Source: CAD feature listing. Evaluate the final solid. Frame: model axes, mm. A direction names the side the tool comes from. Round coordinates to 2 decimals unless told otherwise and drop trailing zeros. Loops run counter-clockwise (first coordinate to the right, second up) from the corner with the lowest first, then second, coordinate; pieces in that order, holes last. Notation, with made-up numbers: (6.25, 65.25) -> (62.25, 65.25) arc R20 ccw to (62.25, 77.25) -> close; hole circle Ø6 at (32.5, 89). An arc over 180 degrees is marked (long way). Put each result on its own line as item: value. Start each with the question number.
1. Material intervals for L1, parallel to X at y = 98, z = 17; L2, parallel to Y at x = 15, z = 1.2; L3, parallel to Z at x = 19, y = 74, sorted ascending.
2. Set-up query: faces 1 (the cylindrical face through (0, 81, 10)), 2 (the flat face through (22.9, 72.35, 1.48)), 3 (the flat face through (-22.956, 72.567, 1.479)), 4 (the cylindrical face through (20.91, 85.2, 16.48)), 5 (the cylindrical face through (14.979, 108.449, 4.725)). Return all of +Z, -Z, +X, -X, +Y, -Y with unobstructed straight access to the full face (end or side cutting, diameter ignored); none if empty.
3. Cut plane C-C (x = -2.5). State how many separate pieces and enclosed holes the cut face has, then the cut area to 3 significant figures.
4. Draft query along Y for faces 6 (the flat face through (0, 111, 15.5)), 7 (the flat face through (24.547, 78.741, 8.916)), 8 (the cylindrical face through (6.693, 109.541, 7.371)). Return one class per face: pulls with the +Y half, pulls with the -Y half, needs draft (parallel to the pull), parting line crosses it, or undercut.
5. Cut plane B-B (y = 82). Return the cut outline in (x, z).
6. Cut plane A-A (z = 8.25). Return the cut outline in (x, y), then the cut area to 3 significant figures.
7. Contact query for flat-ended pins moving along their axis: pin 1 (8 mm diameter, centred on x = 4, y = 70, fed in from +Z); pin 2 (2.5 mm diameter, centred on x = -0.5, y = 110.5, fed in from +Z); pin 3 (6 mm diameter, centred on x = 0, z = 8.25, fed in from -Y). Output: stop coordinate, or through.
```python
from build123d import *

# Parameters (mm, degrees)
SKETCH1_R                 = 2
BOSS_EXTRUDE1_DEPTH       = 3
BOSS_EXTRUDE2_DEPTH       = 12
SKETCH3_R                 = 1.5
BOSS_EXTRUDE3_DEPTH       = 3
FILLET1_R                 = 10
FILLET3_R                 = 3.5
BOSS_EXTRUDE6_DEPTH       = 14
BOSS_EXTRUDE7_DEPTH       = 0.5
BOSS_EXTRUDE8_START       = -14
BOSS_EXTRUDE8_DEPTH       = 14
FILLET7_R                 = 30
FILLET11_R                = 30
CUT_EXTRUDE3_REACH        = 52.603
CUT_EXTRUDE3_END_RADIUS   = 47
SKETCH12_R                = 3.75
BOSS_EXTRUDE9_REACH       = 64
BOSS_EXTRUDE9_END_RADIUS  = 47
SKETCH13_R                = 6.75
SKETCH13_R_2              = 3.75
BOSS_EXTRUDE10_REACH      = 59.242
BOSS_EXTRUDE10_END_RADIUS = 44
SKETCH14_R                = 6.75
SKETCH14_R_2              = 3.75


# Some blends are built 0.0001 mm under size
with BuildPart() as part:
    # Sketch1 → Boss-Extrude1 (new body)
    with BuildSketch(Plane.XY):
        with BuildLine():
            Line((20.854716842, 64.723108589), (25, 80.193515947))
            ThreePointArc((25, 80.193515947), (0, 84), (-25, 80.193515947))
            Line((-25, 80.193515947), (-20.854716842, 64.723108589))
            ThreePointArc((-20.854716842, 64.723108589), (0, 68), (20.854716842, 64.723108589))
        make_face()
        with Locations((15, 70.420167566)):
            Circle(SKETCH1_R, mode=Mode.SUBTRACT)
        with Locations(Location((-15, 70.420167566, 0), (0, 0, 180))):
            Circle(SKETCH1_R, mode=Mode.SUBTRACT)
    extrude(amount=BOSS_EXTRUDE1_DEPTH)

    # Sketch2 → Boss-Extrude2 (add)
    with BuildSketch(Plane.XY.offset(3)):
        with BuildLine():
            Line((-25, 80.193515947), (-24.107142857, 77.329461806))
            ThreePointArc((-24.107142857, 77.329461806), (0, 81), (24.107142857, 77.329461806))
            Line((24.107142857, 77.329461806), (25, 80.193515947))
            ThreePointArc((25, 80.193515947), (0, 84), (-25, 80.193515947))
        make_face()
    extrude(amount=BOSS_EXTRUDE2_DEPTH)

    # Sketch3 → Boss-Extrude3 (add)
    with BuildSketch(Plane.XY.offset(15)):
        with BuildLine():
            Line((-31.5, 77.329461806), (-31.5, 105.329461806))
            Line((-31.5, 105.329461806), (-24.5, 105.329461806))
            Line((-24.5, 105.329461806), (-24.5, 80.347681983))
            ThreePointArc((-24.5, 80.347681983), (0, 84), (24.5, 80.347681983))
            Line((24.5, 80.347681983), (24.5, 105.329461806))
            Line((24.5, 105.329461806), (31.5, 105.329461806))
            Line((31.5, 105.329461806), (31.5, 77.329461806))
            Line((31.5, 77.329461806), (24.107142857, 77.329461806))
            ThreePointArc((24.107142857, 77.329461806), (0, 81), (-24.107142857, 77.329461806))
            Line((-24.107142857, 77.329461806), (-31.5, 77.329461806))
        make_face()
        with Locations((-28, 101.920167566)):
            Circle(SKETCH3_R, mode=Mode.SUBTRACT)
        with Locations(Location((28, 101.920167566, 0), (0, 0, 180))):
            Circle(SKETCH3_R, mode=Mode.SUBTRACT)
    extrude(amount=BOSS_EXTRUDE3_DEPTH)

    # Fillet1
    # the kernel refuses this fillet: 10 mm, written as the material it adds along each edge
    with BuildSketch(Plane(origin=(24.5, 80.347681983, 15), x_dir=(-0.9747000358663407, 0.22351697940459464, 0), z_dir=(0, 0, 1))) as fillet1_piece_1:
        with BuildLine():
            CenterArc((12.54704984, -9.975125536), FILLET1_R, 94.042076765, 98.87360977)
            Line((2.800049481, -12.21029533), (0, 0))
            ThreePointArc((0, 0), (5.9210797, -0.208945494), (11.8421594, 0))
        make_face()
    extrude(amount=3)
    with BuildSketch(Plane(origin=(-24.5, 80.347681983, 15), x_dir=(0.9747000358663402, 0.22351697940459697, 0), z_dir=(0, 0, 1))) as fillet1_piece_2:
        with BuildLine():
            CenterArc((12.54704984, 9.975125536), FILLET1_R, 167.084313465, 98.87360977)
            Line((2.800049481, 12.21029533), (0, 0))
            ThreePointArc((0, 0), (5.9210797, 0.208945494), (11.8421594, 0))
        make_face()
    extrude(amount=3)
    # the kernel refuses this fillet: 10 mm, written as the material it takes off along each edge
    with BuildSketch(Plane(origin=(31.5, 77.329461806, 15), x_dir=(0, 1, 0), z_dir=(0, 0, 1))) as fillet1_2_piece_1:
        with BuildLine():
            CenterArc((9.654160042, 10), FILLET1_R, 195.112449543, 74.887550457)
            Line((0, 7.392857143), (0, 0))
            Line((0, 0), (9.654160042, 0))
        make_face()
    extrude(amount=27.135400106, mode=Mode.SUBTRACT)
    with BuildSketch(Plane(origin=(-31.5, 77.329461806, 15), x_dir=(0, 1, 0), z_dir=(0, 0, 1))) as fillet1_2_piece_2:
        with BuildLine():
            CenterArc((9.654160042, -10), FILLET1_R, 90, 74.887550457)
            Line((0, -7.392857143), (0, 0))
            Line((0, 0), (9.654160042, 0))
        make_face()
    extrude(amount=27.135400106, mode=Mode.SUBTRACT)

    # Fillet3
    fillet3_edges = [part.edges().sort_by_distance(p)[0] for p in [
        (31.5, 105.329461806, 16.5),
        (24.5, 105.329461806, 16.5),
        (-24.5, 105.329461806, 16.5),
        (-31.5, 105.329461806, 16.5),
    ]]
    fillet(fillet3_edges, radius=FILLET3_R - 0.0001)  # a hair under: the kernel refuses the full size



with BuildPart() as body_2:
    # Sketch9 → Boss-Extrude6 (new body)
    with BuildSketch(Plane(origin=(0, 0, 15), x_dir=(-1, 0, 0), z_dir=(0, 0, -1))):
        with BuildLine():
            ThreePointArc((24.654911386, 102.8592104), (0, 110.415619131), (-24.654911386, 102.8592104))
            ThreePointArc((-24.654911386, 102.8592104), (-25.431275444, 104.2067826), (-26.71481938, 105.084966494))
            ThreePointArc((-26.71481938, 105.084966494), (0, 113.415619131), (26.71481938, 105.084966494))
            ThreePointArc((26.71481938, 105.084966494), (25.431275444, 104.2067826), (24.654911386, 102.8592104))
        make_face()
    extrude(amount=BOSS_EXTRUDE6_DEPTH)


with BuildPart() as part_1:
    add(part.part)

    add(body_2.part)  # Boss-Extrude7 merges body 2
    # Sketch10 → Boss-Extrude7 (add)
    with BuildSketch(Plane.XY.offset(15)):
        with BuildLine():
            ThreePointArc((-24.654911386, 102.8592104), (-25.431275444, 104.2067826), (-26.71481938, 105.084966494))
            ThreePointArc((-26.71481938, 105.084966494), (0, 113.415619131), (26.71481938, 105.084966494))
            ThreePointArc((26.71481938, 105.084966494), (25.431275444, 104.2067826), (24.654911386, 102.8592104))
            ThreePointArc((24.654911386, 102.8592104), (0, 110.415619131), (-24.654911386, 102.8592104))
        make_face()
    extrude(amount=BOSS_EXTRUDE7_DEPTH)

    # Sketch11 → Boss-Extrude8 (add)
    with BuildSketch(Plane(origin=(0, 0, 1), x_dir=(-1, 0, 0), z_dir=(0, 0, -1)).offset(BOSS_EXTRUDE8_START)):
        with BuildLine():
            Line((-26.71481938, 105.084966494), (-24.654911386, 102.8592104))
            ThreePointArc((-24.654911386, 102.8592104), (-25.431275444, 104.2067826), (-26.71481938, 105.084966494))
        make_face()
        with BuildLine():
            Line((26.71481938, 105.084966494), (24.654911386, 102.8592104))
            ThreePointArc((24.654911386, 102.8592104), (25.431275444, 104.2067826), (26.71481938, 105.084966494))
        make_face()
    extrude(amount=BOSS_EXTRUDE8_DEPTH)

    # Fillet7
    # the kernel refuses this fillet: 30 mm, written as the material it takes off along each edge
    with BuildSketch(Plane(origin=(69.80741828, 151.647053217, 1), x_dir=(-0.7339213016528682, 0.6792345125066597, 0), z_dir=(-0.6792345125066598, -0.7339213016528682, 0))) as fillet7_piece_1_section:
        with BuildLine():
            CenterArc((25.377155081, -30), FILLET7_R, 90, 57.769047365)
            Line((0, -14), (0, 0))
            Line((0, 0), (25.377155081, 0))
        make_face()
    fillet7_piece_1 = extrude(amount=129.918465817, mode=Mode.PRIVATE)
    fillet7_piece_1 = fillet7_piece_1 - Plane(origin=(0, 0, 1), x_dir=(0.2976190476190481, 0.9546847136590859, 0), z_dir=(0, 0, -1)) * Cylinder(84, 362, mode=Mode.PRIVATE)
    add(fillet7_piece_1, mode=Mode.SUBTRACT)
    with BuildSketch(Plane(origin=(-69.80741828, 151.647053217, 1), x_dir=(0, 0, 1), z_dir=(0.6792345125066636, -0.7339213016528646, 0))) as fillet7_piece_2_section:
        with BuildLine():
            CenterArc((30, -25.377155081), FILLET7_R, 122.230952636, 57.769047365)
            Line((0, -25.377155081), (0, 0))
            Line((0, 0), (14, 0))
        make_face()
    fillet7_piece_2 = extrude(amount=129.918465817, mode=Mode.PRIVATE)
    fillet7_piece_2 = fillet7_piece_2 - Plane(origin=(0, 0, 1), x_dir=(0.2976190476190481, 0.9546847136590859, 0), z_dir=(0, 0, -1)) * Cylinder(84, 362, mode=Mode.PRIVATE)
    add(fillet7_piece_2, mode=Mode.SUBTRACT)

    # Fillet11
    # the kernel refuses this fillet: 30 mm, written as the material it adds along each edge
    with BuildSketch(Plane(origin=(27.9999, 101.829561806, 15.5), x_dir=(0.5609336863803128, 0.8278607367690491, 0), z_dir=(0.8278607367690491, -0.5609336863803128, 0))) as fillet11_piece_1_section:
        with BuildLine():
            CenterArc((15.489478808, 30), FILLET11_R, 246.443535691, 23.556464309)
            Line((3.4999, 2.5), (3.4999, 0))
            Line((3.4999, 0), (15.489478808, 0))
        make_face()
    fillet11_piece_1 = revolve(axis=Axis((27.9999, 101.829561806, 15.5), (0, 0, 1)), revolution_arc=359.64, mode=Mode.PRIVATE)
    fillet11_piece_1 = fillet11_piece_1 & Plane(origin=(0, 66.415619131, 15.5), x_dir=(0.5684004123362708, 0.8227520715598091, 0), z_dir=(0, 0, 1)) * Cylinder(47, 62, mode=Mode.PRIVATE)
    fillet11_piece_1 = fillet11_piece_1 - Plane(origin=(0, 66.415619131, 15.5), x_dir=(-0.5603388951384309, 0.8282634379199909, 0), z_dir=(0, 0, 1)) * Cylinder(44, 62, mode=Mode.PRIVATE)
    fillet11_piece_1 = split(fillet11_piece_1, bisect_by=Plane(origin=(31.5, 101.829561806, 15.5), z_dir=(-1, 0, 0)), keep=Keep.TOP, mode=Mode.PRIVATE)
    add(fillet11_piece_1)
    with BuildSketch(Plane(origin=(-27.9999, 101.829561806, 15.5), x_dir=(-0.5661241822221539, 0.8243199684001945, 0), z_dir=(0.8243199684001945, 0.5661241822221539, 0))) as fillet11_piece_2_section:
        with BuildLine():
            CenterArc((15.489478808, 30), FILLET11_R, 246.443535691, 23.556464309)
            Line((3.4999, 2.5), (3.4999, 0))
            Line((3.4999, 0), (15.489478808, 0))
        make_face()
    fillet11_piece_2 = revolve(axis=Axis((-27.9999, 101.829561806, 15.5), (0, 0, 1)), revolution_arc=359.64, mode=Mode.PRIVATE)
    fillet11_piece_2 = fillet11_piece_2 & Plane(origin=(0, 66.415619131, 15.5), x_dir=(0.5684004123362708, 0.8227520715598091, 0), z_dir=(0, 0, 1)) * Cylinder(47, 62, mode=Mode.PRIVATE)
    fillet11_piece_2 = fillet11_piece_2 - Plane(origin=(0, 66.415619131, 15.5), x_dir=(-0.5603388951384309, 0.8282634379199909, 0), z_dir=(0, 0, 1)) * Cylinder(44, 62, mode=Mode.PRIVATE)
    fillet11_piece_2 = split(fillet11_piece_2, bisect_by=Plane(origin=(-31.5, 101.829561806, 15.5), z_dir=(1, 0, 0)), keep=Keep.TOP, mode=Mode.PRIVATE)
    add(fillet11_piece_2)

    # Cut-Extrude3: up to this cylinder (the profile starts inside it)
    cut_extrude3_end = Plane(origin=(0, 66.415619131, 8.250105), z_dir=(0, 0, -1)) * Cylinder(CUT_EXTRUDE3_END_RADIUS, 200.206, mode=Mode.PRIVATE)
    # Sketch12 → Cut-Extrude3 (cut, up to the surface)
    with BuildSketch(Plane(origin=(0, 100, 0), x_dir=(1, 0, 0), z_dir=(0, 1, 0)), mode=Mode.PRIVATE) as cut_extrude3_sk1:
        with Locations(Location((0, -8.250104745, 0), (0, 0, 90))):
            Circle(SKETCH12_R)
    cut_extrude3_tool1 = extrude(cut_extrude3_sk1.sketch, amount=CUT_EXTRUDE3_REACH, mode=Mode.PRIVATE) & cut_extrude3_end
    add(cut_extrude3_tool1.solids().sort_by_distance((0, 100, 8.250105))[0], mode=Mode.SUBTRACT)

    # Boss-Extrude9: up to this cylinder (the profile starts outside it)
    boss_extrude9_end = Plane(origin=(0, 66.415619131, 1.691024), z_dir=(0, 0, -1)) * Cylinder(BOSS_EXTRUDE9_END_RADIUS, 223, mode=Mode.PRIVATE)
    # Sketch13 → Boss-Extrude9 (add, up to the surface)
    with BuildSketch(Plane(origin=(0, 115, 0), x_dir=(1, 0, 0), z_dir=(0, 1, 0)), mode=Mode.PRIVATE) as boss_extrude9_sk1:
        with Locations(Location((0, -8.250104745, 0), (0, 0, 270))):
            Circle(SKETCH13_R)
        with Locations(Location((0, -8.250104745, 0), (0, 0, 90))):
            Circle(SKETCH13_R_2, mode=Mode.SUBTRACT)
    boss_extrude9_tool1 = extrude(boss_extrude9_sk1.sketch, amount=-BOSS_EXTRUDE9_REACH, mode=Mode.PRIVATE) - boss_extrude9_end
    add(boss_extrude9_tool1.solids().sort_by_distance((0, 115, 1.691024))[0])

    # Boss-Extrude10: up to this cylinder (the profile starts inside it)
    boss_extrude10_end = Plane(origin=(0, 66.415619131, 1.691024), z_dir=(0, 0, -1)) * Cylinder(BOSS_EXTRUDE10_END_RADIUS, 207.484, mode=Mode.PRIVATE)
    # Sketch14 → Boss-Extrude10 (add, up to the surface)
    with BuildSketch(Plane(origin=(0, 109, 0), x_dir=(1, 0, 0), z_dir=(0, 1, 0)), mode=Mode.PRIVATE) as boss_extrude10_sk1:
        with Locations(Location((0, -8.250104745, 0), (0, 0, 270))):
            Circle(SKETCH14_R)
        with Locations(Location((0, -8.250104745, 0), (0, 0, 270))):
            Circle(SKETCH14_R_2, mode=Mode.SUBTRACT)
    boss_extrude10_tool1 = extrude(boss_extrude10_sk1.sketch, amount=BOSS_EXTRUDE10_REACH, mode=Mode.PRIVATE) & boss_extrude10_end
    add(boss_extrude10_tool1.solids().sort_by_distance((0, 109, 1.691024))[0])


solid = part_1.part
```
Solution:
1. L1: x = -31.5 to -24.5, 24.5 to 31.5
1. L2: y = 66.32 to 68.42, 72.42 to 82.65
1. L3: z = 0 to 3
2. face 1: +Z, -Y
2. face 2: -Z, +X, -Y
2. face 3: -Z, -X, -Y
2. face 4: +Z, -Z
2. face 5: -Z, +X
3. separate pieces: 3
3. enclosed holes: 0
3. area: 140 mm^2
4. face 6: needs draft
4. face 7: pulls with the -Y half
4. face 8: undercut
5. outline: (-30.17, 15) -> (-18.22, 15) -> (-18.22, 0) -> (18.22, 0) -> (18.22, 15) -> (30.17, 15) -> (30.17, 18) -> (-30.17, 18) -> close
6. outline: (-25, 80.19) -> (-24.11, 77.33) arc R81 cw to (24.11, 77.33) -> (25, 80.19) arc R84 ccw to start; (-21.62, 108.15) -> (-19.5, 105.86) arc R44 cw to (-6.75, 109.89) -> (-6.75, 109) -> (-3.75, 109) -> (-3.75, 115) -> (-6.75, 115) -> (-6.75, 112.93) arc R47 ccw to start; (3.75, 109) -> (6.75, 109) -> (6.75, 109.89) arc R44 cw to (19.5, 105.86) -> (21.62, 108.15) arc R47 ccw to (6.75, 112.93) -> (6.75, 115) -> (3.75, 115) -> close
6. area: 273 mm^2
7. pin 1: stops at z = 3
7. pin 2: stops at z = 15.5
7. pin 3: stops at y = 80.94
